For this review, take the finished solid that the model builds, in its own axes (mm). A direction names the side the tool comes from. Round coordinates to 2 decimals unless told otherwise and drop trailing zeros. Order: outer loops, then holes, each group sorted by start corner. A loop starts at its lowest first (then second) coordinate and runs counter-clockwise, first axis right, second up. Notation, with made-up numbers: (-19.75, 20.5) -> (12.25, 20.5) arc R24 cw to (12.25, 51.5) -> close; hole circle Ø10 at (34.25, 21). An arc over 180 degrees is marked (long way). Use a Markdown table: item, result. Add a question column.
1) Consider section A-A (y = -2.5). Give the number of separate pieces and of enclosed holes in the cut face, plus the area to 3 significant figures.
2) Machinability: for faces 4 (the face through (34.737, -3.757, 34.426)), 5 (the face through (68.58, -4, 214)), 6 (the face through (129, 0, 30)), which of the approach directions +Z, -Z, +X, -X, +Y, -Y give a long, thin tool a straight path to every point of the face, cutting with its end or side? Answer none if there is none.
3) Clearance check with a flat-ended pin moving along its axis: P1, Ø4, axis at x = 116, y = -2, coming from the +Z side. State where the tip first meets the part, or that it passes through.
4) Consider section B-B (z = 166). State the section outline as (x, y) points (3 decimals).
5) Draft analysis for pull direction Z (two halves, no side actions). For faces 1 (the face through (34.93, -3.76, 194.37)), 2 (the face through (3.82, -6.26, 224.98)), 3 (the face through (300.98, -6.26, 3.62)), state which applies: pulls with the +Z half, pulls with the -Z half, needs draft (parallel to the pull), parting line crosses it, or undercut.
6) Wall thickness on line 1 along X through (y, z) = (-3, 215.9); line 2 along Z through (x, y) = (12.7, -9.75); line 3 along Z through (x, y) = (292.1, -5): over which ranges is each line inside the solid? List them lowest first. Write a range as [from, to].
```python
from build123d import *

# Parameters (mm, degrees)
F0_R     = 1.5875
F1_DEPTH = 12.7
F3_DEPTH = 7.62
F4_W     = 196.85
F4_H     = 147.828
F4_R     = 1.5875
F5_DEPTH = 25.4


with BuildPart() as f1:
    # F0 (on Front) → F1 (new body)
    with BuildSketch(Plane.XZ):
        with BuildLine():
            Line((292.1, 228.6), (12.7, 228.6))
            ThreePointArc((12.7, 228.6), (3.719744, 224.880256), (0, 215.9))
            Line((0, 215.9), (0, 12.7))
            ThreePointArc((0, 12.7), (3.719744, 3.719744), (12.7, 0))
            Line((12.7, 0), (292.1, 0))
            ThreePointArc((292.1, 0), (301.080256, 3.719744), (304.8, 12.7))
            Line((304.8, 12.7), (304.8, 215.9))
            ThreePointArc((304.8, 215.9), (301.080256, 224.880256), (292.1, 228.6))
        make_face()
        with Locations((12.7, 12.7)):
            Circle(F0_R, mode=Mode.SUBTRACT)
        with Locations((292.1, 12.7)):
            Circle(F0_R, mode=Mode.SUBTRACT)
        with Locations((12.7, 215.9)):
            Circle(F0_R, mode=Mode.SUBTRACT)
        with Locations((292.1, 215.9)):
            Circle(F0_R, mode=Mode.SUBTRACT)
    extrude(amount=F1_DEPTH)

    # F2 (on face) → F3 (cut)
    with BuildSketch(Plane.XZ):
        with BuildLine():
            ThreePointArc((31.115, 43.307), (34.834744, 34.326744), (43.815, 30.607))
            Line((43.815, 30.607), (260.985, 30.607))
            ThreePointArc((260.985, 30.607), (269.965256, 34.326744), (273.685, 43.307))
            Line((273.685, 43.307), (273.685, 107.95))
            Line((273.685, 107.95), (304.8, 107.95))
            Line((304.8, 107.95), (304.8, 120.65))
            Line((304.8, 120.65), (273.685, 120.65))
            Line((273.685, 120.65), (273.685, 185.293))
            ThreePointArc((273.685, 185.293), (269.965256, 194.273256), (260.985, 197.993))
            Line((260.985, 197.993), (119.38, 197.993))
            Line((119.38, 197.993), (119.38, 228.6))
            Line((119.38, 228.6), (68.58, 228.6))
            Line((68.58, 228.6), (68.58, 197.993))
            Line((68.58, 197.993), (43.815, 197.993))
            ThreePointArc((43.815, 197.993), (34.834744, 194.273256), (31.115, 185.293))
            Line((31.115, 185.293), (31.115, 43.307))
        make_face()
    extrude(amount=F3_DEPTH, mode=Mode.SUBTRACT)

    # F4 (on face) → F5 (cut)
    with BuildSketch(Plane.XZ):
        with Locations((152.4, 114.3)):
            Rectangle(F4_W, F4_H)
        with BuildLine():
            Line((266.7, 109.855), (266.7, 118.745))
            ThreePointArc((266.7, 118.745), (265.39809, 121.88809), (262.255, 123.19))
            ThreePointArc((262.255, 123.19), (259.11191, 121.88809), (257.81, 118.745))
            Line((257.81, 118.745), (257.81, 109.855))
            ThreePointArc((257.81, 109.855), (259.11191, 106.71191), (262.255, 105.41))
            ThreePointArc((262.255, 105.41), (265.39809, 106.71191), (266.7, 109.855))
        make_face()
        with Locations((292.1, 215.9)):
            Circle(F4_R)
        with Locations((12.7, 215.9)):
            Circle(F4_R)
        with Locations((12.7, 12.7)):
            Circle(F4_R)
        with Locations((292.1, 12.7)):
            Circle(F4_R)
    extrude(amount=F5_DEPTH, mode=Mode.SUBTRACT)


solid = f1.part
```
Results list:
| question | item | result |
|---|---|---|
| 1 | separate pieces | 2 |
| 1 | enclosed holes | 4 |
| 1 | area | 27,100 mm2 |
| 2 | face 4 | +Y |
| 2 | face 5 | +Z, +Y |
| 2 | face 6 | +Z, -Z, +X, -X, +Y |
| 3 | P1 | z = 30.61 |
| 4 | outline | (0, -12.7) -> (53.975, -12.7) -> (53.975, -7.62) -> (31.115, -7.62) -> (31.115, 0) -> (0, 0) -> close; (250.825, -12.7) -> (304.8, -12.7) -> (304.8, 0) -> (273.685, 0) -> (273.685, -7.62) -> (250.825, -7.62) -> close |
| 5 | face 1 | undercut |
| 5 | face 2 | pulls with the +Z half |
| 5 | face 3 | pulls with the -Z half |
| 6 | line 1 | [0, 11.11], [14.29, 68.58], [119.38, 290.51], [293.69, 304.8] |
| 6 | line 2 | [0, 11.11], [14.29, 214.31], [217.49, 228.6] |
| 6 | line 3 | [0, 11.11], [14.29, 107.95], [120.65, 214.31], [217.49, 228.6] |
